```python
from build123d import *

# Parameters (mm, degrees)
CROQUIS1_R              = 3.5
CROQUIS1_W              = 8
CROQUIS1_H              = 8
SALIENTE_EXTRUIR1_DEPTH = 3


with BuildPart() as part:
    # Croquis1 → Saliente-Extruir1 (new body)
    with BuildSketch(Plane.XY):
        with BuildLine():
            Line((-10, 0), (-7.5, -45))
            ThreePointArc((-7.5, -45), (0, -52.5), (7.5, -45))
            Line((7.5, -45), (10, 0))
            ThreePointArc((10, 0), (0, 10), (-10, 0))
        make_face()
        with Locations((0, -45)):
            Circle(CROQUIS1_R, mode=Mode.SUBTRACT)
        Rectangle(CROQUIS1_W, CROQUIS1_H, mode=Mode.SUBTRACT)
    extrude(amount=SALIENTE_EXTRUIR1_DEPTH)


solid = part.part
```
The listing builds one solid part. Answer for the finished solid, in the listing's coordinates (mm). A direction names the side the tool comes from. Coordinates: 2 decimals unless noted, no trailing zeros. Loops run counter-clockwise (first coordinate to the right, second up) from the corner with the lowest first, then second, coordinate; pieces in that order, holes last. Notation, with made-up numbers: (-18, 31) - (-13, 31) arc R21 cw to (-13, 42) - close; hole circle Ø5 at (-14, 64). An arc over 180 degrees is marked (long way). Write item = value, one per line.
1) Section B-B (z = 1.75) is taken. Determine the outline of the cut face in (x, y), plus the area to 3 significant figures.
Responses:
outline = (-10, 0) - (-7.5, -45) arc R7.5 ccw to (7.5, -45) - (10, 0) arc R10 ccw to start; hole (-4, -4) - (4, -4) - (4, 4) - (-4, 4) - close; hole circle Ø7 at (0, -45)
area = 930 mm^2
2) Section C-C (y = -43) is taken. Determine the outline of the cut face in (x, z), plus the area to 3 significant figures.
Responses:
outline = (-7.61, 0) - (-2.87, 0) - (-2.87, 3) - (-7.61, 3) - close; (2.87, 0) - (7.61, 0) - (7.61, 3) - (2.87, 3) - close
area = 28.4 mm^2
3) Determine the mould class of faces 1 (the face through (-4, 0, 1)), 2 (the face through (-8.768, -22.185, 1.479)), 3 (the face through (0, -21, 3)), 4 (the face through (-0.46, -41.53, 1.48)) for opening direction Y: pulls with the +Y half, pulls with the -Y half, needs draft (parallel to the pull), parting line crosses it, or undercut.
Responses:
face_1 = undercut
face_2 = pulls with the -Y half
face_3 = needs draft
face_4 = undercut
4) Section A-A (x = 0) is taken. Determine the outline of the cut face in (y, z).
Responses:
outline = (-52.5, 0) - (-48.5, 0) - (-48.5, 3) - (-52.5, 3) - close; (-41.5, 0) - (-4, 0) - (-4, 3) - (-41.5, 3) - close; (4, 0) - (10, 0) - (10, 3) - (4, 3) - close
5) Find the intervals of material crossed by line 1 along Y through (x, z) = (0, 1.8); line 2 along Y through (x, z) = (1.5, 0.5); line 3 along X through (y, z) = (1, 2.05), in increasing order.
Responses:
line_1 = -52.5 to -48.5, -41.5 to -4, 4 to 10
line_2 = -52.35 to -48.16, -41.84 to -4, 4 to 9.89
line_3 = -9.95 to -4, 4 to 9.95
6) Each of these flat-tipped pins is pushed along its axis until it touches: P1, Ø2, axis at x = -6.5, y = -14, coming from the -Z side; P2, Ø1.5, axis at y = 2, z = 2.5, coming from the -X side; P3, Ø4, axis at x = 0, y = -45, coming from the -Z side. Where does it stop, or does it pass through?
Responses:
P1 = 0
P2 = -9.92
P3 = through
7) Section D-D (y = -18) is taken. Determine the outline of the cut face in (x, z).
Responses:
outline = (-9, 0) - (9, 0) - (9, 3) - (-9, 3) - close
8) Which of the six approach directions +Z, -Z, +X, -X, +Y, -Y give full straight-line access (tool end or side, diameter ignored) to faces 5 (the face through (0, 10, 1)), 6 (the face through (0, -4, 1))?
Responses:
face_5 = +Z, -Z, +Y
face_6 = +Z, -Z
